from build123d import *

# Parameters (mm, degrees)
SKETCH1_R           = 9
BOSS_EXTRUDE1_DEPTH = 35
SKETCH2_R           = 10.726971326
SKETCH2_R_2         = 7.95
CUT_EXTRUDE1_DEPTH  = 33
FILLET1_R           = 1
SKETCH3_R           = 6.418564364
CUT_EXTRUDE2_DEPTH  = 1
SKETCH4_W           = 0.5
SKETCH4_H           = 2.354367894
CUT_EXTRUDE3_DEPTH  = 1


with BuildPart() as part:
    # Sketch1 → Boss-Extrude1 (new body)
    with BuildSketch(Plane.XY):
        Circle(SKETCH1_R)
    extrude(amount=BOSS_EXTRUDE1_DEPTH)

    # Sketch2 → Cut-Extrude1 (cut)
    with BuildSketch(Plane(origin=(0, 0, 0), x_dir=(-1, 0, 0), z_dir=(0, 0, -1))):
        Circle(SKETCH2_R)
        Circle(SKETCH2_R_2, mode=Mode.SUBTRACT)
    extrude(amount=-CUT_EXTRUDE1_DEPTH, mode=Mode.SUBTRACT)

    # Fillet1
    fillet1_edges = [part.edges().sort_by_distance(p)[0] for p in [
        (-9, 0, 35),
    ]]
    fillet(fillet1_edges, radius=FILLET1_R)

    # Sketch3 → Cut-Extrude2 (cut)
    with BuildSketch(Plane.XY.offset(35)):
        Circle(SKETCH3_R)
    extrude(amount=-CUT_EXTRUDE2_DEPTH, mode=Mode.SUBTRACT)

    # Sketch4 → Cut-Extrude3 (cut)
    with BuildSketch(Plane.XY.offset(34)):
        with BuildLine():
            Line((-3.395267389, 3.395267389), (-3.041713998, 3.041713998))
            ThreePointArc((-3.041713998, 3.041713998), (0, -4.301633189), (3.041713998, 3.041713998))
            Line((3.041713998, 3.041713998), (3.395267389, 3.395267389))
            ThreePointArc((3.395267389, 3.395267389), (0, -4.801633189), (-3.395267389, 3.395267389))
        make_face()
        with Locations((0, 4.302029464)):
            Rectangle(SKETCH4_W, SKETCH4_H)
    extrude(amount=-CUT_EXTRUDE3_DEPTH, mode=Mode.SUBTRACT)


solid = part.part
Could you check a few things on this model? Use its own coordinates, in mm. A direction names the side the tool comes from. Round coordinates to 2 decimals unless told otherwise and drop trailing zeros. Write each loop counter-clockwise with the first axis right and the second up, starting at its lowest first coordinate (ties: lowest second). Pieces come first, ordered by that corner, then holes. Notation, with made-up numbers: (89, 43.5) - (95, 43.5) arc R33 ccw to (95, 82.5) - close; hole circle Ø2 at (53.5, -33). An arc over 180 degrees is marked (long way). Use a Markdown table: item, result.
Q1. I want a section at A-A (y = 0). List the corners of the cut face in (x, z) for me.
Output values:
| item | result |
|---|---|
| outline | (-9, 33) - (-7.95, 33) - (-7.95, 0) - (7.95, 0) - (7.95, 33) - (9, 33) - (9, 34) arc R1 ccw to (8, 35) - (6.42, 35) - (6.42, 34) - (4.8, 34) - (4.8, 33) - (4.3, 33) - (4.3, 34) - (-4.3, 34) - (-4.3, 33) - (-4.8, 33) - (-4.8, 34) - (-6.42, 34) - (-6.42, 35) - (-8, 35) arc R1 ccw to (-9, 34) - close |
Q2. For faces 4 (the flat face through (-5, -7, 33)), 5 (the flat face through (0.25, 4.3, 33.5)), 6 (the flat face through (0, 0, 0)), which set-ups out of +Z, -Z, +X, -X, +Y, -Y let a thin tool reach every point of the face, with its end or its side?
Output values:
| item | result |
|---|---|
| face 4 | -Z |
| face 5 | +Z |
| face 6 | -Z, +X, -X, +Y, -Y |
Q3. Please list where these lines run through material, in increasing order: L1, parallel to X at y = 0, z = 33.75; L2, parallel to Y at x = 0, z = 33.8; L3, parallel to Z at x = 3.25, y = -0.75.
Output values:
| item | result |
|---|---|
| L1 | -9 to -4.8, -4.3 to 4.3, 4.8 to 9 |
| L2 | -9 to -4.8, -4.3 to 3.12, 5.48 to 9 |
| L3 | 0 to 34 |
Q4. I want a section at B-B (z = 25). List the corners of the cut face in (x, y) for me, plus the area to 3 significant figures.
Output values:
| item | result |
|---|---|
| outline | circle Ø15.9 at (0, 0) |
| area | 199 mm2 |
Q5. For pin 1 (5 mm diameter, centred on y = 6.5, z = 7.5, fed in from -X); pin 2 (1 mm diameter, centred on x = -5.5, z = 20.5, fed in from -Y); pin 3 (2 mm diameter, centred on x = 2.5, y = -2, fed in from +Z), each with a flat end and sliding along its axis, tell me the tip position at first contact or that it passes through.
Output values:
| item | result |
|---|---|
| pin 1 | x = -6.87 |
| pin 2 | y = -6.18 |
| pin 3 | z = 34 |
Q6. Thinking about a two-plate mould opening in Y: for faces 1 (the cylindrical face through (1.72, -7.76, 16.27)), 2 (the flat face through (0, 7, 35)), 3 (the flat face through (1.09, -4.33, 33)), which applies, released by +Y, released by -Y, zero draft, split by the parting line, or undercut?
Output values:
| item | result |
|---|---|
| face 1 | split by the parting line |
| face 2 | zero draft |
| face 3 | undercut |
